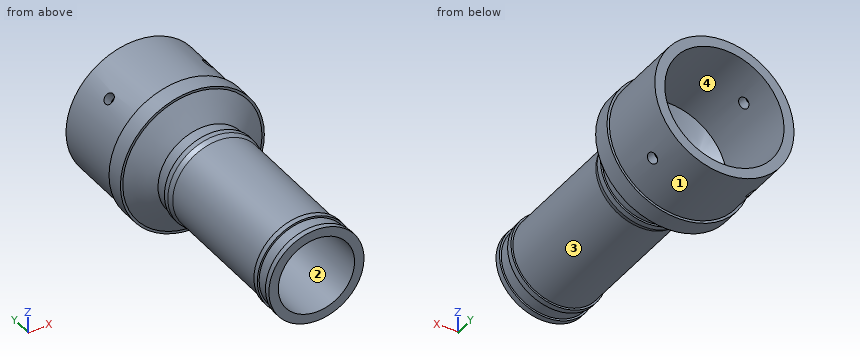
```python
from build123d import *

# Parameters (mm, degrees)
SKETCH2_R                 = 25
SKETCH2_R_2               = 20.85
BOSS_EXTRUDE1_DEPTH       = 99.25
BOSS_EXTRUDE2_START       = 10
SKETCH3_R                 = 38.05
SKETCH3_R_2               = 32.6
BOSS_EXTRUDE2_DEPTH       = 50
BOSS_EXTRUDE3_START       = -50
BOSS_EXTRUDE3_OUTLINE_R   = 39.35
BOSS_EXTRUDE3_OUTLINE_R_2 = 38.05
BOSS_EXTRUDE3_DEPTH       = 10
CUT_EXTRUDE1_REACH        = 186.77
CUT_EXTRUDE1_END_RADIUS   = 32.6
SKETCH7_R                 = 3
CIRPATTERN1_COUNT         = 4
SKETCH8_R                 = 26
SKETCH8_R_2               = 25
BOSS_EXTRUDE5_DEPTH       = 3
BOSS_EXTRUDE6_START       = -92.05
BOSS_EXTRUDE6_OUTLINE_R   = 26
BOSS_EXTRUDE6_OUTLINE_R_2 = 25
BOSS_EXTRUDE6_DEPTH       = 6
CHAMFER1_SIZE             = 1.091910703
CHAMFER1_SIZE_2           = 3
BOSS_EXTRUDE7_START       = -10.2
SKETCH10_R                = 26
SKETCH10_R_2              = 25
BOSS_EXTRUDE7_DEPTH       = 3


with BuildPart() as part:
    # Sketch2 → Boss-Extrude1 (new body)
    with BuildSketch(Plane(origin=(0, 0, 0), x_dir=(1, 0, 0), z_dir=(0, 1, 0))):
        with Locations(Location((0, 0, 0), (0, 0, 270))):
            Circle(SKETCH2_R)
        with Locations(Location((0, 0, 0), (0, 0, 270))):
            Circle(SKETCH2_R_2, mode=Mode.SUBTRACT)
    extrude(amount=BOSS_EXTRUDE1_DEPTH)



with BuildPart() as body_2:
    # Sketch3 → Boss-Extrude2 (new body)
    with BuildSketch(Plane(origin=(0, 99.25, 0), x_dir=(1, 0, 0), z_dir=(0, 1, 0)).offset(BOSS_EXTRUDE2_START)):
        with Locations(Location((0, 0, 0), (0, 0, 270))):
            Circle(SKETCH3_R)
        with Locations(Location((0, 0, 0), (0, 0, 270))):
            Circle(SKETCH3_R_2, mode=Mode.SUBTRACT)
    extrude(amount=BOSS_EXTRUDE2_DEPTH)


with BuildPart() as part_1:
    add(part.part)

    add(body_2.part)  # loft3 joins it to this body
    # loft up to a face of the part (loft3)
    loft([Face(Wire([part_1.edges().sort_by_distance((18.224215686, 99.25, -17.113677648))[0]])), Face(Wire([part_1.edges().sort_by_distance((-27.737256273, 109.25, -26.047017381))[0]]))])

    # Cut-Loft1: read off the stored shape, not the designer's step
    # Cut-Loft1: loft between two sections, ruled curve by curve
    cut_loft1_from = [
        Edge.make_bspline([(-19.857674291, 99.25, 6.355727475), (-7.146219341, 99.25, 46.071076058), (32.569129241, 99.25, 33.359621108), (19.857674291, 99.25, -6.355727475), (7.146219341, 99.25, -46.071076058), (-32.569129241, 99.25, -33.359621108), (-19.857674291, 99.25, 6.355727475)], [0, 0, 0, 0, 0.5, 0.5, 0.5, 1, 1, 1, 1], 3, [1, 0.333333333, 0.333333333, 1, 0.333333333, 0.333333333, 1]),
    ]
    cut_loft1_to = [
        Edge.make_bspline([(-21.296342667, 109.25, 24.682499651), (28.068656636, 109.25, 67.275184984), (70.661341969, 109.25, 17.910185682), (21.296342667, 109.25, -24.682499651), (-28.068656636, 109.25, -67.275184984), (-70.661341969, 109.25, -17.910185682), (-21.296342667, 109.25, 24.682499651)], [0, 0, 0, 0, 0.5, 0.5, 0.5, 1, 1, 1, 1], 3, [1, 0.333333333, 0.333333333, 1, 0.333333333, 0.333333333, 1]),
    ]
    cut_loft1 = Solid(Shell([*[Face.make_surface_from_curves(cut_loft1_from[k], cut_loft1_to[k]) for k in range(1)], Face(Wire(cut_loft1_from)), Face(Wire(cut_loft1_to))]))
    add(cut_loft1, mode=Mode.SUBTRACT)

    # Boss-Extrude3: read off the stored shape, not the designer's step
    # Boss-Extrude3 outline → Boss-Extrude3 (add)
    with BuildSketch(Plane(origin=(0, 159.25, 0), x_dir=(1, 0, 0), z_dir=(0, 1, 0)).offset(BOSS_EXTRUDE3_START)):
        Circle(BOSS_EXTRUDE3_OUTLINE_R)
        Circle(BOSS_EXTRUDE3_OUTLINE_R_2, mode=Mode.SUBTRACT)
    extrude(amount=BOSS_EXTRUDE3_DEPTH)

    # Cut-Extrude1: up to this cylinder (the profile starts outside it)
    cut_extrude1_end = Plane(origin=(0, 139.25, 0), z_dir=(0, -1, 0)) * Cylinder(CUT_EXTRUDE1_END_RADIUS, 439.74, mode=Mode.PRIVATE)
    # Sketch7 → Cut-Extrude1 (cut, up to the surface)
    with BuildSketch(Plane(origin=(-26.905413024, 0, 26.905413024), x_dir=(0, -1, 0), z_dir=(-0.7071067811865488, 0, 0.7071067811865464)), mode=Mode.PRIVATE) as cut_extrude1_sk1:
        with Locations(Location((-139.25, 0, 0), (0, 0, 90))):
            Circle(SKETCH7_R)
    cut_extrude1_tool1 = extrude(cut_extrude1_sk1.sketch, amount=-CUT_EXTRUDE1_REACH, mode=Mode.PRIVATE) - cut_extrude1_end
    cut_extrude1 = cut_extrude1_tool1.solids().sort_by_distance((-26.905413, 139.25, 26.905413))[0]
    add(cut_extrude1, mode=Mode.SUBTRACT)

    # CirPattern1: Cut-Extrude1 ×4 about axis
    cirpattern1_axis = Axis((0, 159.25, 0), (0, -1, 0))
    for i in range(1, CIRPATTERN1_COUNT):
        add(cut_extrude1.rotate(cirpattern1_axis, i * 360 / CIRPATTERN1_COUNT), mode=Mode.SUBTRACT)

    # Sketch8 → Boss-Extrude5 (add)
    with BuildSketch(Plane.XZ):
        with Locations(Location((0, 0, 0), (0, 0, 270))):
            Circle(SKETCH8_R)
        with Locations(Location((0, 0, 0), (0, 0, 270))):
            Circle(SKETCH8_R_2, mode=Mode.SUBTRACT)
    extrude(amount=-BOSS_EXTRUDE5_DEPTH)

    # Boss-Extrude6: read off the stored shape, not the designer's step
    # Boss-Extrude6 outline → Boss-Extrude6 (add)
    with BuildSketch(Plane.XZ.offset(BOSS_EXTRUDE6_START)):
        Circle(BOSS_EXTRUDE6_OUTLINE_R)
        Circle(BOSS_EXTRUDE6_OUTLINE_R_2, mode=Mode.SUBTRACT)
    extrude(amount=BOSS_EXTRUDE6_DEPTH)

    # Chamfer1
    # the kernel refuses this chamfer: 3, 1.091910703 mm, written as the material it takes off along each edge
    with BuildSketch(Plane(origin=(0, 86.05, 0), x_dir=(1, 0, 0), z_dir=(0, 0, -1))) as chamfer1_piece_1_section:
        Polygon((26 - CHAMFER1_SIZE, 0), (26, -CHAMFER1_SIZE_2), (26, 0), align=None)
    chamfer1_piece_1 = revolve(axis=Axis((0, 86.05, 0), (0, -1, 0)), mode=Mode.PRIVATE)
    chamfer1_piece_1 = chamfer1_piece_1 - Plane(origin=(0, 86.05, 0), x_dir=(0, 0, 1), z_dir=(0, -1, 0)) * Cylinder(25, 104, mode=Mode.PRIVATE)
    add(chamfer1_piece_1, mode=Mode.SUBTRACT)

    # Sketch10 → Boss-Extrude7 (add)
    with BuildSketch(Plane.XZ.offset(BOSS_EXTRUDE7_START)):
        with Locations(Location((0, 0, 0), (0, 0, 270))):
            Circle(SKETCH10_R)
        with Locations(Location((0, 0, 0), (0, 0, 270))):
            Circle(SKETCH10_R_2, mode=Mode.SUBTRACT)
    extrude(amount=-BOSS_EXTRUDE7_DEPTH)


solid = part_1.part
```
Can you work these out from the model? Positions are in its coordinate system, mm. Face numbers are marked on the shaded views. A direction names the side the tool comes from. Coordinates: 2 decimals unless noted, no trailing zeros. Loops run counter-clockwise (first coordinate to the right, second up) from the corner with the lowest first, then second, coordinate; pieces in that order, holes last.
Item 1: I'm going to push flat-ended pins straight in: pin 1 (2 mm diameter, centred on x = 8, y = 79, fed in from +Z); pin 2 (6 mm diameter, centred on x = -21.5, y = 111.5, fed in from +Z); pin 3 (15.5 mm diameter, centred on x = 4.5, z = -9, fed in from -Y); pin 4 (23.5 mm diameter, centred on x = -2.5, z = 18.5, fed in from -Y). Where does each tip first touch, or does it pass through?
Answers below:
pin 1: stops at z = 24
pin 2: stops at z = 34.73
pin 3: passes through
pin 4: stops at y = 0
Item 2: Please list where these lines run through material, in increasing order: L1, parallel to Z at x = 0, y = 127.5; L2, parallel to X at y = 32, z = 0; L3, parallel to Y at x = -12.5, z = -22.5.
Answers below:
L1: z = -38.05 to -32.6, 32.6 to 38.05
L2: x = -25 to -20.85, 20.85 to 25
L3: y = 0 to 3, 10.2 to 13.2, 88.33 to 92.05, 99.82 to 104.22
Item 3: Suppose I cut it at A-A (y = 68.5). Please give me the cut outline in (x, z).
Answers below:
outline: circle Ø50 at (0, 0); hole circle Ø41.7 at (0, 0)
Item 4: Which directions (+Z, -Z, +X, -X, +Y, -Y) give clear straight access to the entire face, cutting with the end or side of a thin tool? Please do the marked faces 3 and 4.
Answers below:
face 3: none
face 4: +Y
Item 5: If we mould it in two halves opening along X, with no side actions, what happens to the marked faces 1 and 2? For each: released by +X, released by -X, zero draft, split by the parting line, or undercut.
Answers below:
face 1: split by the parting line
face 2: undercut
